from build123d import *

# Parameters (mm, degrees)
SKETCH_1_W          = 37.6
SKETCH_1_H          = 28
SKETCH_1_R          = 1.9
EXTRUDE_1_DEPTH     = 27.6
SKETCH_2_R          = 1.9
SKETCH_2_W          = 2.4
SKETCH_2_H          = 10
CUT_EXTRUDE_1_DEPTH = 55.401470568


with BuildPart() as part:
    # 草图1 → 凸台-拉伸1 (new body)
    with BuildSketch(Plane.XY):
        with Locations((18.8, 14)):
            Rectangle(SKETCH_1_W, SKETCH_1_H)
        with Locations(Location((4, 24, 0), (0, 0, 180))):
            Circle(SKETCH_1_R, mode=Mode.SUBTRACT)
        with Locations(Location((33.6, 24, 0), (0, 0, 180))):
            Circle(SKETCH_1_R, mode=Mode.SUBTRACT)
        with Locations(Location((33.6, 4, 0), (0, 0, 180))):
            Circle(SKETCH_1_R, mode=Mode.SUBTRACT)
        with Locations(Location((4, 4, 0), (0, 0, 180))):
            Circle(SKETCH_1_R, mode=Mode.SUBTRACT)
    extrude(amount=EXTRUDE_1_DEPTH)

    # 草图2 → 切除-拉伸1 (cut, through all)
    with BuildSketch(Plane(origin=(37.6, 0, 0), x_dir=(0, 0, -1), z_dir=(1, 0, 0))):
        with Locations(Location((-23.6, 9, 0), (0, 0, 90))):
            Circle(SKETCH_2_R)
        with Locations(Location((-4, 9, 0), (0, 0, 90))):
            Circle(SKETCH_2_R)
        with Locations((-15.8, 5)):
            Rectangle(SKETCH_2_W, SKETCH_2_H)
    extrude(amount=-CUT_EXTRUDE_1_DEPTH, mode=Mode.SUBTRACT)


solid = part.part
Design review of the part built by this model. Coordinates are the model's own, in mm. A direction names the side the tool comes from. Give positions to 0.01 mm unless a question says otherwise; leave off trailing zeros. Order: outer loops, then holes, each group sorted by start corner. A loop starts at its lowest first (then second) coordinate and runs counter-clockwise, first axis right, second up.
1. Add section B-B, the plane y = 4. State the section outline as (x, z) points, then the cut area to 3 significant figures.
Solution:
outline: (0, 0) - (2.1, 0) - (2.1, 14.6) - (0, 14.6) - close; (0, 17) - (2.1, 17) - (2.1, 27.6) - (0, 27.6) - close; (5.9, 0) - (31.7, 0) - (31.7, 14.6) - (5.9, 14.6) - close; (5.9, 17) - (31.7, 17) - (31.7, 27.6) - (5.9, 27.6) - close; (35.5, 0) - (37.6, 0) - (37.6, 14.6) - (35.5, 14.6) - close; (35.5, 17) - (37.6, 17) - (37.6, 27.6) - (35.5, 27.6) - close
area: 756 mm2
2. Add section D-D, the plane y = 9. State the section outline as (x, z) points, then the cut area to 3 significant figures.
Solution:
outline: (0, 0) - (37.6, 0) - (37.6, 2.1) - (0, 2.1) - close; (0, 5.9) - (37.6, 5.9) - (37.6, 14.6) - (0, 14.6) - close; (0, 17) - (37.6, 17) - (37.6, 21.7) - (0, 21.7) - close; (0, 25.5) - (37.6, 25.5) - (37.6, 27.6) - (0, 27.6) - close
area: 662 mm2
3. Tool access review of faces 1 (the flat face through (19, 5, 17)), 2 (the flat face through (19, 14, 27.6)): name each direction out of +Z, -Z, +X, -X, +Y, -Y from which nothing blocks a thin tool from reaching the whole face with its end or side.
Solution:
face 1: +X, -X, -Y
face 2: +Z, +X, -X, +Y, -Y
4. For pin 1 Ø5 at (y, z) = (9.5, 11) entering from -X; pin 2 Ø1.2 at (x, z) = (20, 15.5) entering from -Y, all flat-tipped, find the tip position at first contact; note any pin that passes through.
Solution:
pin 1: stops at x = 0
pin 2: stops at y = 10
5. To check wall thickness, follow L1, parallel to X at y = 24, z = 11; L2, parallel to Y at x = 33.6, z = 20.75; L3, parallel to Z at x = 22, y = 6.25. State the ranges of each line that lie inside material, in increasing order.
Solution:
L1: x = 0 to 2.1, 5.9 to 31.7, 35.5 to 37.6
L2: y = 0 to 2.1, 5.9 to 22.1, 25.9 to 28
L3: z = 0 to 14.6, 17 to 27.6
6. Add section C-C, the plane z = 13. State the section outline as (x, y) points, then the cut area to 3 significant figures.
Solution:
outline: (0, 0) - (37.6, 0) - (37.6, 28) - (0, 28) - close; hole circle Ø3.8 at (4, 4); hole circle Ø3.8 at (4, 24); hole circle Ø3.8 at (33.6, 4); hole circle Ø3.8 at (33.6, 24)
area: 1,010 mm2
7. Add section A-A, the plane x = 4. State the section outline as (y, z) points, then the cut area to 3 significant figures.
Solution:
outline: (0, 0) - (2.1, 0) - (2.1, 14.6) - (0, 14.6) - close; (0, 17) - (2.1, 17) - (2.1, 27.6) - (0, 27.6) - close; (5.9, 0) - (22.1, 0) - (22.1, 27.6) - (5.9, 27.6) - (5.9, 17) - (10, 17) - (10, 14.6) - (5.9, 14.6) - close; (25.9, 0) - (28, 0) - (28, 27.6) - (25.9, 27.6) - close; hole circle Ø3.8 at (9, 4); hole circle Ø3.8 at (9, 23.6)
area: 525 mm2
8. Mouldability with a two-part tool opening along X and no side actions: class faces 3 (the flat face through (37.6, 14, 14)), 4 (the flat face through (0, 14, 14)), 5 (the cylindrical face through (31.788, 23.429, 13.607)), 6 (the flat face through (19, 10, 16)) as +X half, -X half, draft (parallel to the pull), parting line (faces both ways), or undercut.
Solution:
face 3: +X half
face 4: -X half
face 5: undercut
face 6: draft
